from build123d import *

# Parameters (mm, degrees)
F0_W     = 59.587501
F0_H     = 74.550004
F0_W_2   = 54.1
F0_H_2   = 69.45
F1_DEPTH = 15
F2_W     = 59.587501
F2_H     = 74.550004
F3_DEPTH = 3
F4_W     = 10.931132
F4_H     = 15
F5_DEPTH = 5.0369


with BuildPart() as f1:
    # F0 (on Top) → F1 (new body)
    with BuildSketch(Plane.XY):
        with Locations((7.48125, -14.700002)):
            Rectangle(F0_W, F0_H)
        with Locations((8.4, -14.747789)):
            Rectangle(F0_W_2, F0_H_2, mode=Mode.SUBTRACT)
    extrude(amount=F1_DEPTH)

    # F2 (on face) → F3 (join)
    with BuildSketch(Plane(origin=(0, 0, 0), x_dir=(1, 0, 0), z_dir=(0, 0, -1))):
        with Locations((7.48125, 14.700002)):
            Rectangle(F2_W, F2_H)
    extrude(amount=-F3_DEPTH)

    # F4 (on face) → F5 (cut)
    with BuildSketch(Plane(origin=(0, 22.575, 0), x_dir=(-1, 0, 0), z_dir=(0, 1, 0))):
        with Locations((-22.809435, 7.5)):
            Rectangle(F4_W, F4_H)
    extrude(amount=-F5_DEPTH, mode=Mode.SUBTRACT)


solid = f1.part
Build history of the part. All positions in model axes, mm. A direction names the side the tool comes from. Give positions to 0.01 mm unless a question says otherwise; leave off trailing zeros. Write each loop counter-clockwise with the first axis right and the second up, starting at its lowest first coordinate (ties: lowest second). Pieces come first, ordered by that corner, then holes. Notation, with made-up numbers: (-9, -2.5) - (21, -2.5) arc R6 cw to (21, 6.5) - close; hole circle Ø9 at (89, -11.5). An arc over 180 degrees is marked (long way). Use one line per item in the form item = value. Start each with the question number.
1. 3-axis set-ups, long thin cutter, end or side, ignore diameter. For faces 5 (the face through (7, -14, 0)), 6 (the face through (17.344, 21, 6)), 7 (the face through (-18.65, -15, 9)): which of +Z, -Z, +X, -X, +Y, -Y reach the whole face in a straight line?
2. Probe line 1 (Y direction, x = -4, z = 5.5) (3 decimals); line 2 (Z direction, x = -2, y = -32.5); line 3 (Y direction, x = 22.5, z = 6.25) (3 decimals). List the from-to ranges inside material, lowest first. Write a range as [from, to].
3. Drop flat-ended pins along their axis: pin 1 Ø1.5 at (x, y) = (-1, -38.5) entering from +Z; pin 2 Ø3.5 at (x, z) = (24.5, 1.5) entering from +Y. Give the stop position or say it passes through.
4. Band-saw the part on B-B on x = 6. Write the cut outline in (y, z) (3 decimals).
5. Band-saw the part on D-D on x = 24. Write the cut outline in (y, z) (3 decimals).
6. Two-plate mould, pull along X, no slides. Class faces 1 (the face through (-22.313, -15, 7)), 2 (the face through (33, 22.575, 7)), 3 (the face through (8, -49.473, 9)), 4 (the face through (37.275, -15, 7)): released by +X, released by -X, zero draft, split by the parting line, or undercut.
Conclusion:
q1.face_5 = -Z, +X, -X, +Y, -Y
q1.face_6 = +Z, -Z, +Y
q1.face_7 = +Z
q2.line_1 = [-51.975, -49.473], [19.977, 22.575]
q2.line_2 = [0, 3]
q2.line_3 = [-51.975, -49.473]
q3.pin_1 = 3
q3.pin_2 = 17.54
q4.outline = (-51.975, 0) - (22.575, 0) - (22.575, 15) - (19.977, 15) - (19.977, 3) - (-49.473, 3) - (-49.473, 15) - (-51.975, 15) - close
q5.outline = (-51.975, 0) - (17.538, 0) - (17.538, 3) - (-49.473, 3) - (-49.473, 15) - (-51.975, 15) - close
q6.face_1 = released by -X
q6.face_2 = zero draft
q6.face_3 = undercut
q6.face_4 = released by +X
